Geometry check sheet. Reference: the model listing, model coordinates, mm. A direction names the side the tool comes from. Coordinates: 2 decimals unless noted, no trailing zeros. Write each loop counter-clockwise with the first axis right and the second up, starting at its lowest first coordinate (ties: lowest second). Pieces come first, ordered by that corner, then holes.
from build123d import *

# Parameters (mm, degrees)
PROFIL_BASE_W                                      = 150
PROFIL_BASE_H                                      = 75
BASE_DEPTH                                         = 10
PROFIL_CYLINDRE_R                                  = 20
CYLINDRE_DEPTH                                     = 10
CONG_1_R                                           = 5
PER_AGE_CENTRAL_D                                  = 30
CHAMBRAGE_POUR_VIS_T_TE_RONDE_BOMB_E_M_D           = 3.4
CHAMBRAGE_POUR_VIS_T_TE_RONDE_BOMB_E_M_CBORE_D     = 7
CHAMBRAGE_POUR_VIS_T_TE_RONDE_BOMB_E_M_CBORE_DEPTH = 2.4
R_P_TITION_LIN_AIRE1_COUNT                         = 5
R_P_TITION_LIN_AIRE1_PITCH                         = 32.5
R_P_TITION_LIN_AIRE1_COUNT_DIR2                    = 3
R_P_TITION_LIN_AIRE1_PITCH_DIR2                    = 27.5


with BuildPart() as part:
    # Profil Base → Base (new body)
    with BuildSketch(Plane(origin=(0, 0, 0), x_dir=(1, 0, 0), z_dir=(0, 1, 0))):
        Rectangle(PROFIL_BASE_W, PROFIL_BASE_H)
    extrude(amount=BASE_DEPTH)

    # Profil Cylindre → Cylindre (add)
    with BuildSketch(Plane(origin=(0, 10, 0), x_dir=(1, 0, 0), z_dir=(0, 1, 0))):
        with Locations(Location((0, 0, 0), (0, 0, 270))):
            Circle(PROFIL_CYLINDRE_R)
    extrude(amount=CYLINDRE_DEPTH)

    # Congé1
    cong_1_edges = [part.edges().sort_by_distance(p)[0] for p in [
        (0, 20, -20),
        (75, 5, 37.5),
        (-75, 5, 37.5),
        (-75, 5, -37.5),
        (75, 5, -37.5),
    ]]
    fillet(cong_1_edges, radius=CONG_1_R)

    # Perçage central (through all)
    with Locations(Plane(origin=(0, 20, 0), x_dir=(1, 0, 0), z_dir=(0, 1, 0))):
        with Locations((0, 0)):
            Hole(PER_AGE_CENTRAL_D / 2)

    # Chambrage pour vis à tête ronde bombée M31 (through all)
    with Locations(Plane(origin=(0, 10, 0), x_dir=(1, 0, 0), z_dir=(0, 1, 0))):
        with Locations((-65, 27.5)):
            chambrage_pour_vis_t_te_ronde_bomb_e_m = CounterBoreHole(CHAMBRAGE_POUR_VIS_T_TE_RONDE_BOMB_E_M_D / 2, CHAMBRAGE_POUR_VIS_T_TE_RONDE_BOMB_E_M_CBORE_D / 2, CHAMBRAGE_POUR_VIS_T_TE_RONDE_BOMB_E_M_CBORE_DEPTH)

    # Répétition linéaire1: Chambrage pour vis _ t_te ronde bomb_e M 5 × 3, 3 skipped
    with Locations(*[(i * R_P_TITION_LIN_AIRE1_PITCH, 0, j * R_P_TITION_LIN_AIRE1_PITCH_DIR2) for i in range(R_P_TITION_LIN_AIRE1_COUNT) for j in range(R_P_TITION_LIN_AIRE1_COUNT_DIR2) if (i, j) not in ((0, 0), (1, 1), (2, 1), (3, 1))]):
        add(chambrage_pour_vis_t_te_ronde_bomb_e_m, mode=Mode.SUBTRACT)


solid = part.part
1. Sectioned sample at D-D, the plane x = 0. Record the boundary of the cut face in (y, z).
Computed values:
outline: (0, -37.5) - (10, -37.5) - (10, -31) - (7.6, -31) - (7.6, -29.2) - (0, -29.2) - close; (0, -25.8) - (7.6, -25.8) - (7.6, -24) - (10, -24) - (10, -20) - (15, -20) arc R5 ccw to (20, -15) - (0, -15) - close; (0, 15) - (20, 15) arc R5 ccw to (15, 20) - (10, 20) - (10, 24) - (7.6, 24) - (7.6, 25.8) - (0, 25.8) - close; (0, 29.2) - (7.6, 29.2) - (7.6, 31) - (10, 31) - (10, 37.5) - (0, 37.5) - close
2. Access from +Z, -Z, +X, -X, +Y, -Y to the whole of each face (thin tool, end or side, straight path). Record for faces 1 (the flat face through (-63, 7.6, -28)), 2 (the cylindrical face through (0.221, 3.747, -29.186)).
Computed values:
face 1: +Y
face 2: +Y, -Y
3. Sectioned sample at C-C, the plane z = 0. Record the boundary of the cut face in (x, y), and give its area (3 significant figures).
Computed values:
outline: (-75, 0) - (-66.7, 0) - (-66.7, 7.6) - (-68.5, 7.6) - (-68.5, 10) - (-75, 10) - close; (-63.3, 0) - (-15, 0) - (-15, 20) arc R5 ccw to (-20, 15) - (-20, 10) - (-61.5, 10) - (-61.5, 7.6) - (-63.3, 7.6) - close; (15, 0) - (63.3, 0) - (63.3, 7.6) - (61.5, 7.6) - (61.5, 10) - (20, 10) - (20, 15) arc R5 ccw to (15, 20) - close; (66.7, 0) - (75, 0) - (75, 10) - (68.5, 10) - (68.5, 7.6) - (66.7, 7.6) - close
area: 1,200 mm2
4. Sectioned sample at B-B, the plane y = 2. Give the number of separate pieces and of enclosed holes in the cut face, and give its area (3 significant figures).
Computed values:
separate pieces: 1
enclosed holes: 13
area: 10,400 mm2
5. Sectioned sample at A-A, the plane x = -32.5. Record the boundary of the cut face in (y, z).
Computed values:
outline: (0, -37.5) - (10, -37.5) - (10, -31) - (7.6, -31) - (7.6, -29.2) - (0, -29.2) - close; (0, -25.8) - (7.6, -25.8) - (7.6, -24) - (10, -24) - (10, 24) - (7.6, 24) - (7.6, 25.8) - (0, 25.8) - close; (0, 29.2) - (7.6, 29.2) - (7.6, 31) - (10, 31) - (10, 37.5) - (0, 37.5) - close
6. Gauge pin test, flat ends, axial feed: pin 1 Ø3.5 at (x, z) = (-65, 1) entering from +Y; pin 2 Ø3 at (x, z) = (0, -27.5) entering from -Y; pin 3 Ø11 at (x, z) = (32.5, -27.5) entering from +Y. Record the tip position at first contact, or that the pin passes through.
Computed values:
pin 1: stops at y = 7.6
pin 2: passes through
pin 3: stops at y = 10
7. Thickness scan on line 1 along Z through (x, y) = (0, 4.75); line 2 along X through (y, z) = (4.5, 27.5); line 3 along Z through (x, y) = (-32.5, 2.5). Record the ranges inside material, lowest first.
Computed values:
line 1: z = -37.5 to -29.2, -25.8 to -15, 15 to 25.8, 29.2 to 37.5
line 2: x = -75 to -66.7, -63.3 to -34.2, -30.8 to -1.7, 1.7 to 30.8, 34.2 to 63.3, 66.7 to 75
line 3: z = -37.5 to -29.2, -25.8 to 25.8, 29.2 to 37.5
8. Draft check along Z on faces 3 (the flat face through (-75, 5, 0)), 4 (the cylindrical face through (0, 9, -31)), 5 (the flat face through (-1, 5, -37.5)). Enter one of: released by +Z, released by -Z, zero draft, split by the parting line, or undercut.
Computed values:
face 3: zero draft
face 4: undercut
face 5: released by -Z
